CAD build for the part. Positions are in the model's coordinates, mm. Coordinates: 2 decimals unless noted, no trailing zeros. Loops run counter-clockwise (first coordinate to the right, second up) from the corner with the lowest first, then second, coordinate; pieces in that order, holes last. Notation, with made-up numbers: (9, 48) -> (35, 48) arc R30 cw to (35, 78) -> close; hole circle Ø10 at (3.25, -19.5). An arc over 180 degrees is marked (long way). Write item = value, one per line. Start each with the question number.
(1) Band-saw the part on D-D (x = -16). Write the cut outline in (y, z), and give its area (3 significant figures).
(2) Band-saw the part on B-B (y = 0.55). Count the separate pieces of the cut face and the enclosed holes in it, and give its area (3 significant figures).
(3) Drill centre lines: line 1 (X direction, y = 0.6, z = 0); line 2 (Z direction, x = 0, y = 1.4); line 3 (X direction, y = 1.2, z = -19). Where is each one in solid material? Low to high. Write a range as from..to.
(4) Flat gauge pins, fed straight in: P1, Ø1, axis at x = 0, y = 1, coming from the -Z side; P2, Ø4, axis at x = 5.5, z = -19, coming from the +Y side; P3, Ø1, axis at x = -12, y = 0.5, coming from the +Z side. Where does each tip first touch, or does it go through?
(5) Band-saw the part on A-A (x = 0). Write the cut outline in (y, z).
(6) Band-saw the part on C-C (z = -11.5). Write the cut outline in (x, y).
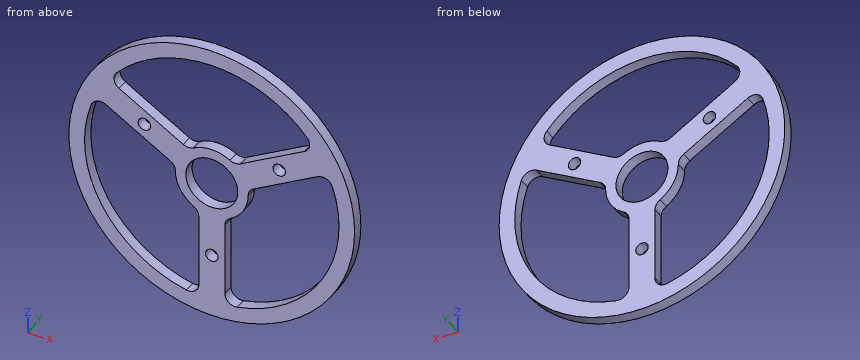
```python
from build123d import *

# Parameters (mm, degrees)
CROQUIS1_R              = 27.5
SALIENTE_EXTRUIR1_DEPTH = 2.11
CROQUIS2_R              = 1.2
CROQUIS2_R_2            = 5
CORTAR_EXTRUIR1_DEPTH   = 3.11
REDONDEO1_R             = 2


with BuildPart() as part:
    # Croquis1 → Saliente-Extruir1 (new body)
    with BuildSketch(Plane(origin=(0, 0, 0), x_dir=(1, 0, 0), z_dir=(0, 1, 0))):
        Circle(CROQUIS1_R)
    extrude(amount=SALIENTE_EXTRUIR1_DEPTH)

    # Croquis2 → Cortar-Extruir1 (cut, through all)
    with BuildSketch(Plane(origin=(0, 2.11, 0), x_dir=(1, 0, 0), z_dir=(0, 1, 0))):
        with Locations((0, 15)):
            Circle(CROQUIS2_R)
        with Locations((12.990381057, -7.5)):
            Circle(CROQUIS2_R)
        with Locations((-12.990381057, -7.5)):
            Circle(CROQUIS2_R)
        Circle(CROQUIS2_R_2)
        with BuildLine():
            Line((-2.5, 6.538348415), (-2.5, 24.372115214))
            ThreePointArc((-2.5, 24.372115214), (-21.217622393, 12.25), (-22.356870919, -10.020994097))
            Line((-22.356870919, -10.020994097), (-6.912375826, -1.104110698))
            ThreePointArc((-6.912375826, -1.104110698), (-6.062177826, 3.5), (-2.5, 6.538348415))
        make_face()
        with BuildLine():
            Line((2.5, 6.538348415), (2.5, 24.372115214))
            ThreePointArc((2.5, 24.372115214), (21.217622393, 12.25), (22.356870919, -10.020994097))
            Line((22.356870919, -10.020994097), (6.912375826, -1.104110698))
            ThreePointArc((6.912375826, -1.104110698), (6.062177826, 3.5), (2.5, 6.538348415))
        make_face()
        with BuildLine():
            Line((4.412375826, -5.434237717), (19.856870919, -14.351121116))
            ThreePointArc((19.856870919, -14.351121116), (0, -24.5), (-19.856870919, -14.351121116))
            Line((-19.856870919, -14.351121116), (-4.412375826, -5.434237717))
            ThreePointArc((-4.412375826, -5.434237717), (0, -7), (4.412375826, -5.434237717))
        make_face()
    extrude(amount=-CORTAR_EXTRUIR1_DEPTH, mode=Mode.SUBTRACT)

    # Redondeo1
    redondeo1_edges = [part.edges().sort_by_distance(p)[0] for p in [
        (-2.5, 1.055, -6.538348415),
        (-6.912375826, 1.055, 1.104110698),
        (-22.356870919, 1.055, 10.020994097),
        (-2.5, 1.055, -24.372115214),
        (-4.412375826, 1.055, 5.434237717),
        (4.412375826, 1.055, 5.434237717),
        (19.856870919, 1.055, 14.351121116),
        (-19.856870919, 1.055, 14.351121116),
        (6.912375826, 1.055, 1.104110698),
        (2.5, 1.055, -6.538348415),
        (2.5, 1.055, -24.372115214),
        (22.356870919, 1.055, 10.020994097),
    ]]
    fillet(redondeo1_edges, radius=REDONDEO1_R)


solid = part.part
```
Findings below:
q1.outline = (0, -22.37) -> (2.11, -22.37) -> (2.11, -18.55) -> (0, -18.55) -> close; (0, 6.35) -> (2.11, 6.35) -> (2.11, 12.12) -> (0, 12.12) -> close; (0, 18.55) -> (2.11, 18.55) -> (2.11, 22.37) -> (0, 22.37) -> close
q1.area = 28.3 mm²
q2.separate_pieces = 1
q2.enclosed_holes = 7
q2.area = 825 mm²
q3.line_1 = -27.5..-24.5, -7..-5, 5..7, 24.5..27.5
q3.line_2 = -27.5..-16.2, -13.8..-5, 5..7, 24.5..27.5
q3.line_3 = -19.88..-15.47, -2.5..2.5, 15.47..19.88
q4.P1 = -27.5
q4.P2 = through
q4.P3 = 24.98
q5.outline = (0, -27.5) -> (2.11, -27.5) -> (2.11, -16.2) -> (0, -16.2) -> close; (0, -13.8) -> (2.11, -13.8) -> (2.11, -5) -> (0, -5) -> close; (0, 5) -> (2.11, 5) -> (2.11, 7) -> (0, 7) -> close; (0, 24.5) -> (2.11, 24.5) -> (2.11, 27.5) -> (0, 27.5) -> close
q6.outline = (-24.98, 0) -> (-21.63, 0) -> (-21.63, 2.11) -> (-24.98, 2.11) -> close; (-2.5, 0) -> (2.5, 0) -> (2.5, 2.11) -> (-2.5, 2.11) -> close; (21.63, 0) -> (24.98, 0) -> (24.98, 2.11) -> (21.63, 2.11) -> close
